Part print with two shaded views. Sizes in mm from the minimum x, y, z corner. A direction names the side the tool comes from. Coordinates: 2 decimals unless noted, no trailing zeros. Loops run counter-clockwise (first coordinate to the right, second up) from the corner with the lowest first, then second, coordinate; pieces in that order, holes last.
Item 1: Drill centre lines: line 1 along Z through (x, y) = (13.5, 9.75); line 2 along Z through (x, y) = (21.75, 6.5); line 3 along Y through (x, z) = (11, 2.95). Where is each one in solid material? Low to high.
Item 2: Flat gauge pins, fed straight in: pin 1 (1.5 mm diameter, centred on y = 4, z = 3, fed in from +X); pin 2 (1 mm diameter, centred on x = 15.5, z = 2.5, fed in from -Y). Where does each tip first touch, or does it go through?
Item 3: Cut at A-A (y = 8.2). List the corners of the cut face in (x, z) (3 decimals).
Item 4: 3-axis set-ups, long thin cutter, end or side, ignore diameter. For the marked faces 1 and 2: which of +Z, -Z, +X, -X, +Y, -Y reach the whole face in a straight line?
Item 5: Cut at C-C (z = 0.7). List the corners of the cut face in (x, y) (3 decimals).
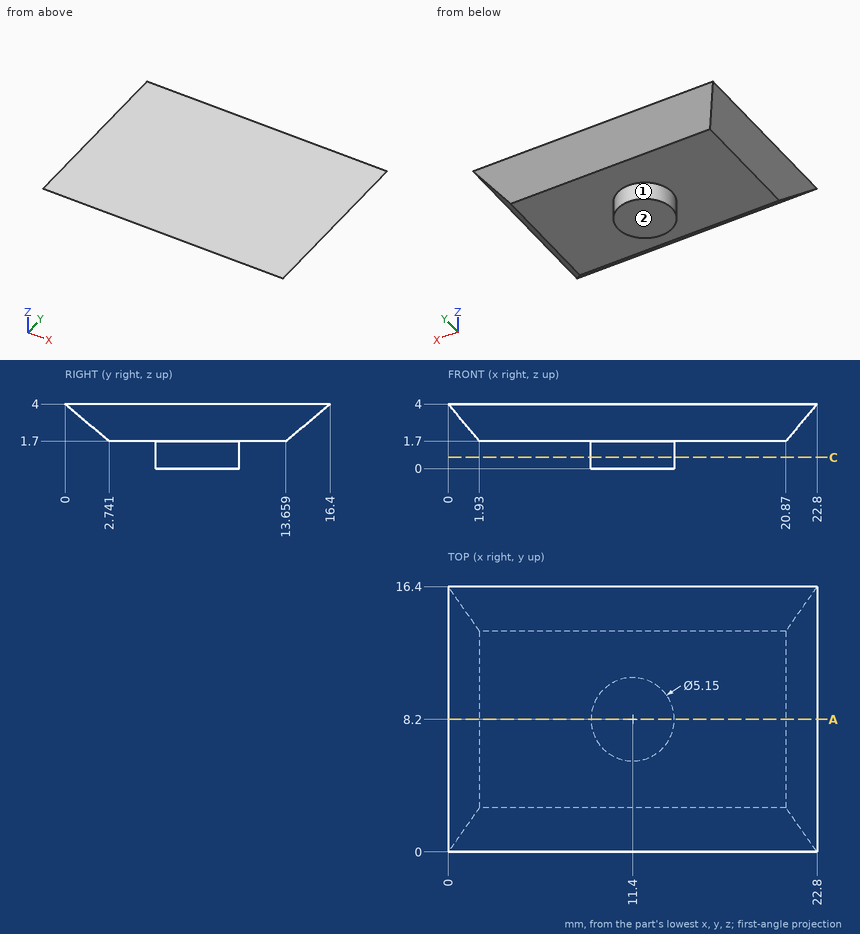
Filled sheet:
1. line 1: z = 1.7 to 4
1. line 2: z = 2.75 to 4
1. line 3: y = 1.25 to 15.15
2. pin 1: stops at x = 22.59
2. pin 2: stops at y = 1.19
3. outline: (0, 4) - (1.93, 1.7) - (8.825, 1.7) - (8.825, 0) - (13.975, 0) - (13.975, 1.7) - (20.87, 1.7) - (22.8, 4) - close
4. face 1: -Z
4. face 2: -Z, +X, -X, +Y, -Y
5. outline: circle Ø5.15 at (11.4, 8.2)
